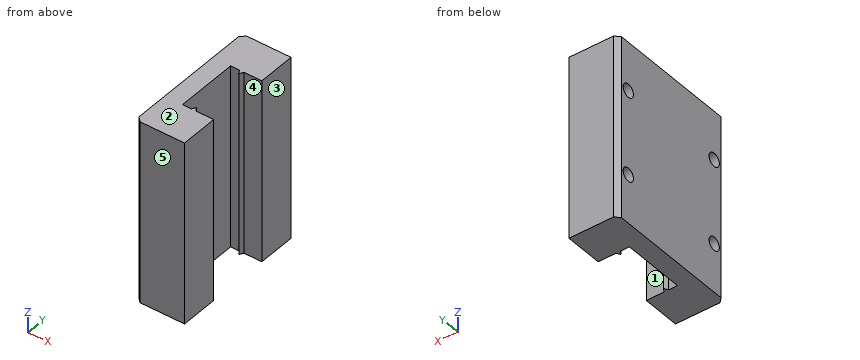
Autodesk Inventor part; units mm, degrees
ref_plane "YZ Plane" through (0, 0, 0) normal (1, 0, 0) x (0, 1, 0)
ref_plane "XZ Plane" through (0, 0, 0) normal (0, 1, 0) x (-1, 0, 0)
ref_plane "XY Plane" through (0, 0, 0) normal (0, 0, 1) x (1, 0, 0)
sketch "Sketch1" plane through (0, 0, 0) normal (0, 0, 1) x (1, 0, 0)
  line L0 (-5.5, -15.5) -> (5.5, -15.5)
  line L1 (5.5, -15.5) -> (5.5, 15.5)
  line L2 (5.5, 15.5) -> (-5.5, 15.5)
  line L3 (-5.5, 15.5) -> (-5.5, -15.5)
  line L4 (0, 0) -> (3.6847, 0)
  line L5 (0, 0) -> (0, -8.9349)
  point P0 (5.5, 0)
  point P1 (0, -15.5)
  dimension "d0" = 11
  dimension "d1" = 31
extrude "Extrusion1" add sketch "Sketch1" along normal blind 41
sketch "Sketch2" plane through (0, 0, 41) normal (0, 0, 1) x (1, 0, 0)
  line L0 (5.5, -15.5) -> (5.5, 15.5)
  line L1 (5.5, -7) -> (-1.5, -7)
  line L2 (-1.5, -7) -> (-1.5, 7)
  line L3 (-1.5, 7) -> (5.5, 7)
  line L4 (5.5, 7) -> (5.5, -7)
  point P0 (0, 0)
  point P1 (5.5, 0)
  dimension "d4" = 7
  dimension "d5" = 14
extrude "Extrusion2" cut sketch "Sketch2" against normal through all
sketch "Sketch3" plane through (0, 0, 41) normal (0, 0, 1) x (1, 0, 0)
  line L0 (-1.5, 7) -> (5.5, 7)
  line L1 (5.5, -7) -> (-1.5, -7)
  line L2 (1, 6.134) -> (0.5, 7)
  line L3 (0.5, 7) -> (-1.5, 7)
  line L4 (-1.5, -7) -> (-1.5, 7)
  line L5 (0.5, -7) -> (-1.5, -7)
  line L6 (0.5, -7) -> (1, -6.134)
  line L7 (1, -6.134) -> (1.5, -7)
  line L8 (7.5, -7) -> (1.5, -7)
  line L9 (7.5, 7) -> (7.5, -7)
  line L10 (7.5, 7) -> (1.5, 7)
  line L11 (1.5, 7) -> (1, 6.134)
  line L12 (0.5, 7) -> (1.5, 7)
  line L13 (1.5, 7) -> (1, 6.134)
  line L14 (1, 6.134) -> (0.5, 7)
  line L15 (1, -6.134) -> (1.5, -7)
  line L16 (1.5, -7) -> (0.5, -7)
  line L17 (0.5, -7) -> (1, -6.134)
  point P0 (0, 0)
  point P1 (1, 6.7113)
  point P2 (1, -6.7113)
  dimension "d8" = 1
  dimension "d9" = 1
  dimension "d10" = 2
  dimension "d11" = 2
extrude "Extrusion3" add sketch "Sketch3" against normal up to surface (41 mm away) contours L0 L11 L2 | L6 L7 L1
sketch "Sketch4" plane through (-5.5, -15.5, 0) normal (-1, 0, 0) x (0, 0, 1)
  line L0 (0, 0) -> (41, 0)
  line L1 (41, 31) -> (41, 0)
  line L2 (0, 31) -> (41, 31)
  circle A0 centre (30, 3) radius 1.5
  line L3 (41, 15.5) -> (23.6881, 15.5)
  line L4 (20.5, 31) -> (20.5, 20.567)
  circle A1 centre (30, 28) radius 1.5
  circle A2 centre (11, 3) radius 1.5
  circle A3 centre (11, 28) radius 1.5
  point P0 (0, 15.5)
  dimension "d14" = 3
  dimension "d15" = 3
  dimension "d16" = 11
extrude "Extrusion4" cut sketch "Sketch4" against normal blind 3
chamfer "Chamfer1" distance 1 angle 45 2 edges at (-5.5, -15.5, 20.5) (-5.5, 15.5, 20.5)
properties part number "Pen_Holder" material "Steel, Wrought"
Build history of the part. All positions in model axes, mm. Face numbers are marked on the shaded views. A direction names the side the tool comes from. Coordinates: 2 decimals unless noted, no trailing zeros. Write each loop counter-clockwise with the first axis right and the second up, starting at its lowest first coordinate (ties: lowest second). Pieces come first, ordered by that corner, then holes.
1. 3-axis set-ups, long thin cutter, end or side, ignore diameter. For the marked faces 1 and 2: which of +Z, -Z, +X, -X, +Y, -Y reach the whole face in a straight line?
Answer block:
face 1: +Z, -Z, +X
face 2: +Z, +X, -X, +Y, -Y
2. Drop flat-ended pins along their axis: pin 1 (1.5 mm diameter, centred on y = 3.5, z = 10.5, fed in from +X); pin 2 (2.5 mm diameter, centred on y = 12.5, z = 11, fed in from -X); pin 3 (2.5 mm diameter, centred on y = -13, z = 10.5, fed in from -X). Give the stop position or say it passes through.
Answer block:
pin 1: stops at x = -1.5
pin 2: stops at x = -2.5
pin 3: stops at x = -5.5
3. Pull direction Y, two halves, no side cores. Call the marked faces 3, 4 and 5: released by +Y, released by -Y, zero draft, split by the parting line, or undercut.
Answer block:
face 3: zero draft
face 4: undercut
face 5: released by -Y
4. Band-saw the part on B-B, the plane y = 12.5. Give the cut face in (x, z), and give its area (3 significant figures).
Answer block:
outline: (-5.5, 0) - (5.5, 0) - (5.5, 41) - (-5.5, 41) - (-5.5, 31.5) - (-2.5, 31.5) - (-2.5, 28.5) - (-5.5, 28.5) - (-5.5, 12.5) - (-2.5, 12.5) - (-2.5, 9.5) - (-5.5, 9.5) - close
area: 433 mm2
5. Drill centre lines: probe 1 along Y at (x, z) = (-4.3, 11); probe 2 along Y at (x, z) = (0, 20); probe 3 along Y at (x, z) = (-4.65, 11). Where is each one in solid material? Low to high.
Answer block:
probe 1: y = -15.5 to -14, -11 to 11, 14 to 15.5
probe 2: y = -15.5 to -7, 7 to 15.5
probe 3: y = -15.35 to -14, -11 to 11, 14 to 15.35
6. Band-saw the part on D-D, the plane z = 30. Give the cut face in (x, y), and give its area (3 significant figures).
Answer block:
outline: (-5.5, -14.5) - (-4.5, -15.5) - (5.5, -15.5) - (5.5, -7) - (1.5, -7) - (1, -6.13) - (0.5, -7) - (-1.5, -7) - (-1.5, 7) - (0.5, 7) - (1, 6.13) - (1.5, 7) - (5.5, 7) - (5.5, 15.5) - (-4.5, 15.5) - (-5.5, 14.5) - (-5.5, 14) - (-2.5, 14) - (-2.5, 11) - (-5.5, 11) - (-5.5, -11) - (-2.5, -11) - (-2.5, -14) - (-5.5, -14) - close
area: 225 mm2
7. Band-saw the part on C-C, the plane z = 14. Give the cut face in (x, y).
Answer block:
outline: (-5.5, -14.5) - (-4.5, -15.5) - (5.5, -15.5) - (5.5, -7) - (1.5, -7) - (1, -6.13) - (0.5, -7) - (-1.5, -7) - (-1.5, 7) - (0.5, 7) - (1, 6.13) - (1.5, 7) - (5.5, 7) - (5.5, 15.5) - (-4.5, 15.5) - (-5.5, 14.5) - close
8. Band-saw the part on A-A, the plane x = 4.25. Give the cut face in (y, z), and give its area (3 significant figures).
Answer block:
outline: (-15.5, 0) - (-7, 0) - (-7, 41) - (-15.5, 41) - close; (7, 0) - (15.5, 0) - (15.5, 41) - (7, 41) - close
area: 697 mm2
